```python
from build123d import *

# Parameters (mm, degrees)
SKETCH_1_W          = 94
SKETCH_1_H          = 58
EXTRUDE_1_DEPTH     = 4
FILLET_1_R          = 3
SKETCH_2_R          = 1.525
CUT_EXTRUDE_1_DEPTH = 10
CUT_EXTRUDE_2_DEPTH = 10
SKETCH_4_R          = 2.025
CUT_EXTRUDE_3_DEPTH = 10
CUT_EXTRUDE_4_DEPTH = 10
FILLET_2_R          = 2
FILLET_3_R          = 3


with BuildPart() as part:
    # 草图1 → 凸台-拉伸1 (new body)
    with BuildSketch(Plane(origin=(0, 0, 0), x_dir=(1, 0, 0), z_dir=(0, 1, 0))):
        Rectangle(SKETCH_1_W, SKETCH_1_H)
    extrude(amount=EXTRUDE_1_DEPTH)

    # 圆角1
    fillet_1_edges = [part.edges().sort_by_distance(p)[0] for p in [
        (47, 2, 29),
        (-47, 2, 29),
        (-47, 2, -29),
        (47, 2, -29),
    ]]
    fillet(fillet_1_edges, radius=FILLET_1_R)

    # 草图2 → 切除-拉伸1 (cut)
    with BuildSketch(Plane(origin=(0, 4, 0), x_dir=(1, 0, 0), z_dir=(0, 1, 0))):
        with Locations((-34.500000003, 5)):
            Circle(SKETCH_2_R)
        with Locations((-34.500000003, -25)):
            Circle(SKETCH_2_R)
        with BuildLine():
            Line((-39.500000003, 14), (-39.500000003, 20))
            ThreePointArc((-39.500000003, 20), (-34.500000003, 25), (-29.500000003, 20))
            Line((-29.500000003, 20), (-29.500000003, 14))
            ThreePointArc((-29.500000003, 14), (-34.500000003, 9), (-39.500000003, 14))
        make_face()
        with BuildLine():
            Line((-39.500000003, -16), (-39.500000003, -4))
            ThreePointArc((-39.500000003, -4), (-34.500000003, 1), (-29.500000003, -4))
            Line((-29.500000003, -4), (-29.500000003, -16))
            ThreePointArc((-29.500000003, -16), (-34.500000003, -21), (-39.500000003, -16))
        make_face()
    cut_extrude_1 = extrude(amount=-CUT_EXTRUDE_1_DEPTH, mode=Mode.SUBTRACT)

    # 镜向1: 切除-拉伸1 across plane
    add(cut_extrude_1.mirror(Plane(origin=(0, 0, 0), x_dir=(0, 0, 1), z_dir=(1, 0, 0))), mode=Mode.SUBTRACT)

    # 草图3 → 切除-拉伸2 (cut)
    with BuildSketch(Plane.XZ):
        Polygon((-22, 29), (-12, 19), (12, 19), (22, 29), align=None)
    cut_extrude_2 = extrude(amount=-CUT_EXTRUDE_2_DEPTH, mode=Mode.SUBTRACT)

    # 镜向2: 切除-拉伸2 across plane
    add(cut_extrude_2.mirror(Plane.XY), mode=Mode.SUBTRACT)

    # 草图4 → 切除-拉伸3 (cut)
    with BuildSketch(Plane.XZ):
        with Locations((0, 5)):
            Circle(SKETCH_4_R)
        with Locations((0, -5)):
            Circle(SKETCH_4_R)
    extrude(amount=-CUT_EXTRUDE_3_DEPTH, mode=Mode.SUBTRACT)

    # 草图5 → 切除-拉伸4 (cut)
    with BuildSketch(Plane.XZ):
        Polygon((-7, 12.5), (-7, -12.5), (-22, 0), align=None)
        Polygon((22, 0), (7, 12.5), (7, -12.5), align=None)
    extrude(amount=-CUT_EXTRUDE_4_DEPTH, mode=Mode.SUBTRACT)

    # 圆角2
    fillet_2_edges = [part.edges().sort_by_distance(p)[0] for p in [
        (-22, 2, 0),
        (-7, 2, 12.5),
        (-7, 2, -12.5),
        (22, 2, 0),
        (7, 2, -12.5),
        (7, 2, 12.5),
    ]]
    fillet(fillet_2_edges, radius=FILLET_2_R)

    # 圆角3
    fillet_3_edges = [part.edges().sort_by_distance(p)[0] for p in [
        (-22, 2, 29),
        (22, 2, 29),
        (12, 2, 19),
        (-12, 2, 19),
        (22, 2, -29),
        (-22, 2, -29),
        (-12, 2, -19),
        (12, 2, -19),
    ]]
    fillet(fillet_3_edges, radius=FILLET_3_R)


solid = part.part
```
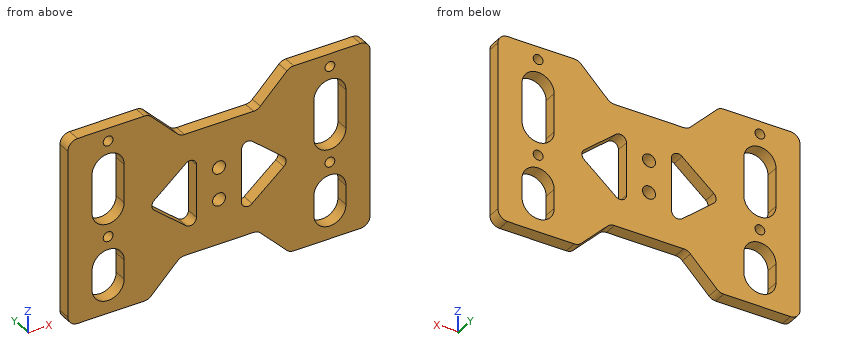
Geometry: final body of the model. Coordinates: model frame, mm. Round coordinates to 2 decimals unless told otherwise and drop trailing zeros. Order: outer loops, then holes, each group sorted by start corner. A loop starts at its lowest first (then second) coordinate and runs counter-clockwise, first axis right, second up. Notation, with made-up numbers: M -17.75,10.5 L 36.25,10.5 A31 ccw 36.25,41.5 Z; hole C 87,31.25 d8. An arc over 180 degrees is marked long. One line per item, written item: value.
(1) Cut plane C-C (z = -5). Return the cut outline in (x, y) (3 decimals), and give its area (3 significant figures).
Result sheet:
outline: M -47,0 L -36.025,0 L -36.025,4 L -47,4 Z; M -32.975,0 L -16,0 L -16,4 L -32.975,4 Z; M -7,0 L -2.025,0 L -2.025,4 L -7,4 Z; M 2.025,0 L 7,0 L 7,4 L 2.025,4 Z; M 16,0 L 32.975,0 L 32.975,4 L 16,4 Z; M 36.025,0 L 47,0 L 47,4 L 36.025,4 Z
area: 263 mm2
(2) Cut plane D-D (x = 34.5). Return the cut outline in (y, z) (3 decimals), and give its area (3 significant figures).
Result sheet:
outline: M 0,-29 L 4,-29 L 4,-25 L 0,-25 Z; M 0,-9 L 4,-9 L 4,-6.525 L 0,-6.525 Z; M 0,-3.475 L 4,-3.475 L 4,-1 L 0,-1 Z; M 0,21 L 4,21 L 4,23.475 L 0,23.475 Z; M 0,26.525 L 4,26.525 L 4,29 L 0,29 Z
area: 55.6 mm2
(3) Pin query (flat end, axial travel): P1, Ø2, axis at x = 4, y = 3, coming from the +Z side; P2, Ø1.8, axis at x = 34.5, z = -5, coming from the +Y side (1 decimal). Return the tip coordinate at first contact, or that it passes through.
Result sheet:
P1: z = 19
P2: through
(4) Cut plane B-B (x = 0). Return the cut outline in (y, z) (3 decimals).
Result sheet:
outline: M 0,-19 L 4,-19 L 4,-7.025 L 0,-7.025 Z; M 0,-2.975 L 4,-2.975 L 4,2.975 L 0,2.975 Z; M 0,7.025 L 4,7.025 L 4,19 L 0,19 Z
(5) Cut plane A-A (z = 25). Return the cut outline in (x, y) (3 decimals), and give its area (3 significant figures).
Result sheet:
outline: M -47,0 L -36.025,0 L -36.025,4 L -47,4 Z; M -32.975,0 L -18,0 L -18,4 L -32.975,4 Z; M 18,0 L 32.975,0 L 32.975,4 L 18,4 Z; M 36.025,0 L 47,0 L 47,4 L 36.025,4 Z
area: 208 mm2
(6) Line query: probe 1 along Z at (x, y) = (0, 2.3) (3 decimals); probe 2 along X at (y, z) = (0.3, -2.5); probe 3 along Z at (x, y) = (34.5, 1.4) (3 decimals). Output: solid intervals per line, ascending. Write a range as [from, to].
Result sheet:
probe 1: [-19, -7.025], [-2.975, 2.975], [7.025, 19]
probe 2: [-47, -19], [-7, 7], [19, 47]
probe 3: [-29, -25], [-9, -6.525], [-3.475, -1], [21, 23.475], [26.525, 29]
